Source: three-view drawing plus pictorial views. Frame: mm from the lowest corner of the part. Give positions to 0.01 mm unless a question says otherwise; leave off trailing zeros. Order: outer loops, then holes, each group sorted by start corner. A loop starts at its lowest first (then second) coordinate and runs counter-clockwise, first axis right, second up. Notation, with made-up numbers: M 77.25,-5.75 L 110.25,-5.75 A20 cw 110.25,29.25 Z; hole C 53.5,-11 d5. An arc over 180 degrees is marked long. Use CSV: the item, a comma, the result in double quotes.
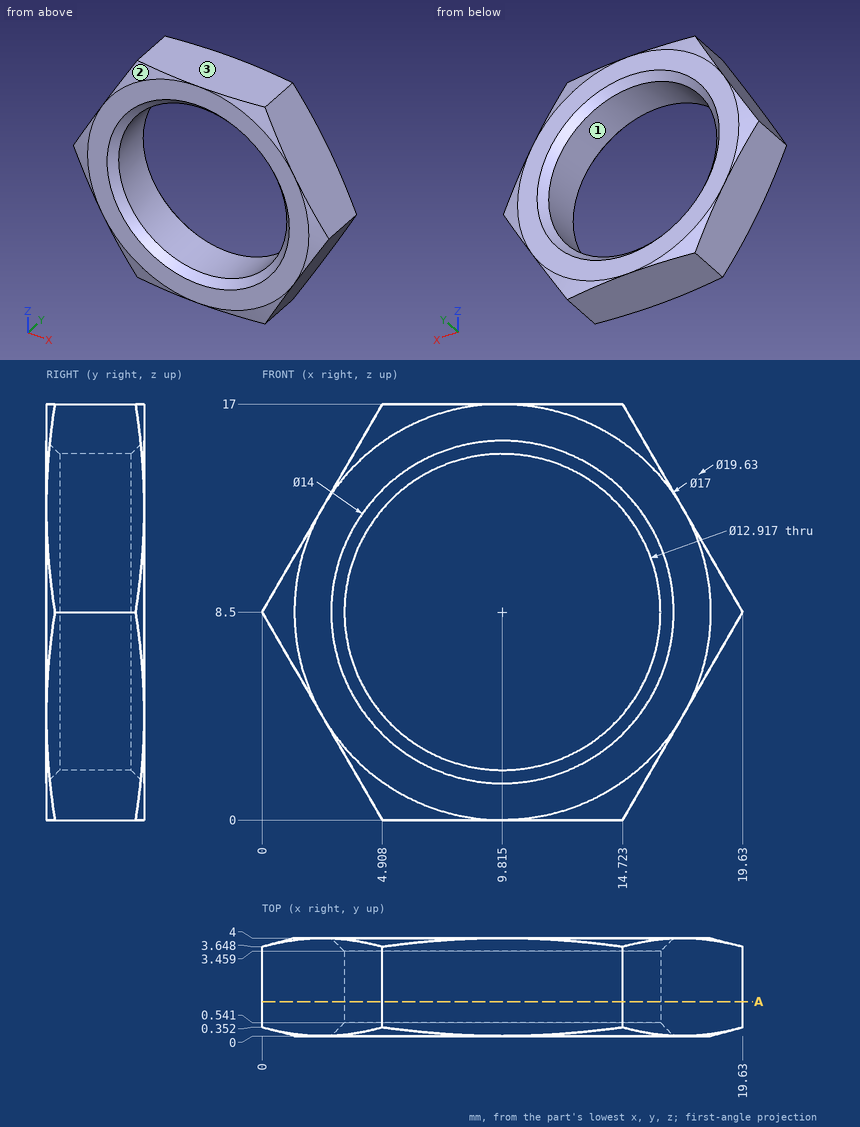
1. Section A-A, the plane y = 1.4. Return the cut outline in (x, z) (1 decimal).
Answer:
outline,"M 0,8.5 L 4.9,0 L 14.7,0 L 19.6,8.5 L 14.7,17 L 4.9,17 Z; hole C 9.8,8.5 d12.9"
2. Line query: line 1 (X direction, y = 2.4, z = 9) (1 decimal); line 2 (X direction, y = 1.8, z = 10) (1 decimal); line 3 (Z direction, x = 10.5, y = 3.6) (1 decimal). Output: solid intervals per line, ascending.
Answer:
line 1,"0.3 to 3.4, 16.3 to 19.3"
line 2,"0.9 to 3.5, 16.1 to 18.8"
line 3,"0 to 1.9, 15.1 to 17"
3. Pin query (flat end, axial travel): pin 1 Ø5 at (x, z) = (12, 14.5) entering from -Y; pin 2 Ø1 at (y, z) = (3, 11.5) entering from -X; pin 3 Ø2 at (y, z) = (3, 10.5) entering from +X. Return the tip coordinate at first contact, or that it passes through.
Answer:
pin 1,"y = 0"
pin 2,"x = 1.44"
pin 3,"x = 19.05"
4. Pull-direction query (Z, two-part tool) for the marked faces 1, 2 and 3; classes: +Z half, -Z half, draft (parallel to the pull), parting line (faces both ways), or undercut.
Answer:
face 1,"undercut"
face 2,"parting line"
face 3,"+Z half"
